```python
from build123d import *

# Parameters (mm, degrees)
SKETCH1_W               = 38.55
SKETCH1_H               = 180
SKETCH1_W_2             = 3.05
SKETCH1_H_2             = 20
SKETCH1_W_3             = 9.833333334
SKETCH1_H_3             = 3
BOSS_EXTRUDE1_DEPTH     = 3
CUT_EXTRUDE4_DEPTH      = 1
CUT_EXTRUDE4_DEPTH_BACK = 4
FILLET1_R               = 2.5


with BuildPart() as part:
    # Sketch1 → Boss-Extrude1 (new body)
    with BuildSketch(Plane.XY):
        Rectangle(SKETCH1_W, SKETCH1_H)
        with Locations((14.75, -20)):
            Rectangle(SKETCH1_W_2, SKETCH1_H_2, mode=Mode.SUBTRACT)
        with Locations((14.75, 20)):
            Rectangle(SKETCH1_W_2, SKETCH1_H_2, mode=Mode.SUBTRACT)
        with Locations((14.75, 60)):
            Rectangle(SKETCH1_W_2, SKETCH1_H_2, mode=Mode.SUBTRACT)
        with Locations((14.75, -60)):
            Rectangle(SKETCH1_W_2, SKETCH1_H_2, mode=Mode.SUBTRACT)
        with Locations((-14.75, 60)):
            Rectangle(SKETCH1_W_2, SKETCH1_H_2, mode=Mode.SUBTRACT)
        with Locations((-14.75, 20)):
            Rectangle(SKETCH1_W_2, SKETCH1_H_2, mode=Mode.SUBTRACT)
        with Locations((-14.75, -20)):
            Rectangle(SKETCH1_W_2, SKETCH1_H_2, mode=Mode.SUBTRACT)
        with Locations((-14.75, -60)):
            Rectangle(SKETCH1_W_2, SKETCH1_H_2, mode=Mode.SUBTRACT)
        with Locations((1.525, -91.5)):
            Rectangle(SKETCH1_W_3, SKETCH1_H_3)
    extrude(amount=BOSS_EXTRUDE1_DEPTH)

    # Sketch3 → Cut-Extrude4 (cut, two sides)
    with BuildSketch(Plane.XY.offset(3)) as cut_extrude4_sk:
        Polygon((2.985254038, 31.119200877), (-5.675, 46.119200877), (2.985254038, 61.119200877), (7.325, 61.119200877), (7.325, 31.119200877), align=None)
        Polygon((2.985254038, -41.626933041), (-5.675, -26.626933041), (2.985254038, -11.626933041), (7.325, -11.626933041), (7.325, -41.626933041), align=None)
        Polygon((-7.175, 67.492267836), (-2.694237886, 67.492267836), (3.372404107, 78), (-7.175, 78), align=None)
        Polygon((-7.175, 24.746133918), (-2.694237886, 24.746133918), (5.966016151, 9.746133918), (-2.694237886, -5.253866082), (-7.175, -5.253866082), align=None)
        Polygon((-7.175, -78), (-7.175, -48), (-2.694237886, -48), (5.966016151, -63), (-2.694237886, -78), align=None)
    extrude(amount=CUT_EXTRUDE4_DEPTH, mode=Mode.SUBTRACT)
    extrude(cut_extrude4_sk.sketch, amount=-CUT_EXTRUDE4_DEPTH_BACK, mode=Mode.SUBTRACT)

    # Fillet1
    fillet1_edges = [part.edges().sort_by_distance(p)[0] for p in [
        (-19.275, 90, 1.5),
        (19.275, 90, 1.5),
    ]]
    fillet(fillet1_edges, radius=FILLET1_R)


solid = part.part
```
Verification items for the finished model (mm, model axes). A direction names the side the tool comes from. Round coordinates to 2 decimals unless told otherwise and drop trailing zeros. Loops run counter-clockwise (first coordinate to the right, second up) from the corner with the lowest first, then second, coordinate; pieces in that order, holes last. Notation, with made-up numbers: (22.25, 68.5) -> (50.25, 68.5) arc R13 ccw to (50.25, 75.5) -> close; hole circle Ø2 at (69.5, 25.25). An arc over 180 degrees is marked (long way). Answer as a JSON object with one key per item and string values.
Q1. Access from +Z, -Z, +X, -X, +Y, -Y to the whole of each face (thin tool, end or side, straight path). Record for faces 1 (the flat face through (4, 0, 3)), 2 (the flat face through (15, -30, 1)).
Data:
{"face 1": "+Z, +X, -X, +Y, -Y", "face 2": "+Z, -Z"}
Q2. Go/stop test with a flat-tipped pin: P1, Ø1.5, axis at x = -15.5, z = 1.5, coming from the -Y side. Record where the tip stops, or that it passes through.
Data:
{"P1": "stops at y = -90"}
Q3. Section check C-C (z = 1.2). State how many separate pieces and enclosed holes the cut face has, then the cut area to 3 significant figures.
Data:
{"separate pieces": "1", "enclosed holes": "13", "area": "5,350 mm2"}
Q4. Scan lines: line 1 (Y direction, x = 16, z = 1.05); line 2 (X direction, y = 27, z = 2.65) (3 decimals); line 3 (Y direction, x = -5.5, z = 2.65). Record each from-to range of solid material in increasing order. Write a range as from..to.
Data:
{"line 1": "y = -90..-70, -50..-30, -10..10, 30..50, 70..90", "line 2": "x = -19.275..-16.275, -13.225..13.225, 16.275..19.275", "line 3": "y = -90..-78, -48..-26.93, -26.32..-5.25, 24.75..45.82, 46.42..67.49, 78..90"}
Q5. Draft check along X on faces 3 (the flat face through (-15, -30, 1)), 4 (the flat face through (-5, 67.492, 2)), 5 (the flat face through (-3.392, -92, 1)), 6 (the flat face through (-11, -90, 1)). Enter one of: pulls with the +X half, pulls with the -X half, needs draft (parallel to the pull), parting line crosses it, or undercut.
Data:
{"face 3": "undercut", "face 4": "undercut", "face 5": "pulls with the -X half", "face 6": "needs draft"}
Q6. Section check A-A (y = 1). Record the boundary of the cut face in (x, z) (3 decimals), then the cut area to 3 significant figures.
Data:
{"outline": "(-19.275, 0) -> (-7.175, 0) -> (-7.175, 3) -> (-19.275, 3) -> close; (0.916, 0) -> (19.275, 0) -> (19.275, 3) -> (0.916, 3) -> close", "area": "91.4 mm2"}
Q7. Section check B-B (y = -24). Record the boundary of the cut face in (x, z) (3 decimals), then the cut area to 3 significant figures.
Data:
{"outline": "(-19.275, 0) -> (-16.275, 0) -> (-16.275, 3) -> (-19.275, 3) -> close; (-13.225, 0) -> (-4.158, 0) -> (-4.158, 3) -> (-13.225, 3) -> close; (7.325, 0) -> (13.225, 0) -> (13.225, 3) -> (7.325, 3) -> close; (16.275, 0) -> (19.275, 0) -> (19.275, 3) -> (16.275, 3) -> close", "area": "62.9 mm2"}
Q8. Section check D-D (y = -68). Record the boundary of the cut face in (x, z) (3 decimals).
Data:
{"outline": "(-19.275, 0) -> (-16.275, 0) -> (-16.275, 3) -> (-19.275, 3) -> close; (-13.225, 0) -> (-7.175, 0) -> (-7.175, 3) -> (-13.225, 3) -> close; (3.079, 0) -> (13.225, 0) -> (13.225, 3) -> (3.079, 3) -> close; (16.275, 0) -> (19.275, 0) -> (19.275, 3) -> (16.275, 3) -> close"}
